Can you work these out from the model? Positions are in its coordinate system, mm. A direction names the side the tool comes from. Coordinates: 2 decimals unless noted, no trailing zeros. Order: outer loops, then holes, each group sorted by start corner. A loop starts at its lowest first (then second) coordinate and runs counter-clockwise, first axis right, second up. Notation, with made-up numbers: M -17,49 L 40,49 A14 cw 40,57 Z; hole C -18,36 d8. An arc over 180 degrees is marked long. Answer as a JSON object with one key per item and string values.
from build123d import *

# Parameters (mm, degrees)
F0_W     = 24
F0_H     = 68
F1_DEPTH = 8
F2_R     = 2
F3_DEPTH = 20
F4_W     = 39.3141321838
F4_H     = 5.4286047816
F4_W_2   = 14.8275513351
F5_DEPTH = 25
F6_W     = 16
F6_H     = 40.9167615801
F6_H_2   = 11.5639846772
F7_DEPTH = 25


with BuildPart() as f1:
    # F0 (on Top) → F1 (new body)
    with BuildSketch(Plane.XY):
        Rectangle(F0_W, F0_H)
    extrude(amount=F1_DEPTH)

    # F2 (on Right) → F3 (join, symmetric)
    with BuildSketch(Plane.YZ):
        with Locations((32, 2)):
            Circle(F2_R)
        with Locations((-15.5, 2)):
            Circle(F2_R)
    extrude(amount=F3_DEPTH, both=True)

    # F4 (on face) → F5 (cut)
    with BuildSketch(Plane.YZ.offset(12)):
        with BuildLine():
            ThreePointArc((30, 8), (32.8284271247, 6.8284271247), (34, 4))
            Line((34, 4), (34, 8))
            Line((34, 8), (30, 8))
        make_face()
        with Locations((7.5888540596, 2.7143023908)):
            Rectangle(F4_W, F4_H)
        with Locations((-26.5862243325, 2.7143023908)):
            Rectangle(F4_W_2, F4_H)
    extrude(amount=-F5_DEPTH, mode=Mode.SUBTRACT)

    # F6 (on face) → F7 (cut)
    with BuildSketch(Plane.XY.offset(8)):
        with Locations((0, 7.775218226)):
            Rectangle(F6_W, F6_H)
        with Locations((0, -25.0811139122)):
            Rectangle(F6_W, F6_H_2)
    extrude(amount=-F7_DEPTH, mode=Mode.SUBTRACT)


solid = f1.part
Item 1: I want a section at A-A, the plane y = 13. Write out the boundary of the cut face in (x, z), plus the area to 3 significant figures.
Answers follow:
{"outline": "M -12,5.43 L -8,5.43 L -8,8 L -12,8 Z; M 8,5.43 L 12,5.43 L 12,8 L 8,8 Z", "area": "20.6 mm^2"}
Item 2: Which directions (+Z, -Z, +X, -X, +Y, -Y) give clear straight access to the entire face, cutting with the end or side of a thin tool? Please do faces 1 (the flat face through (0, 28.234, 4)), 2 (the cylindrical face through (-15.944, 33.847, 1.234)), 3 (the flat face through (3, -32, 5.429)).
Answers follow:
{"face 1": "+Z, -Z", "face 2": "-X", "face 3": "-Z, +X, -X, -Y"}
Item 3: I want a section at D-D, the plane x = 9.5. Write out the boundary of the cut face in (y, z).
Answers follow:
{"outline": "M -34,5.43 L -19.17,5.43 L -19.17,0 L -12.07,0 L -12.07,5.43 L 27.25,5.43 L 27.25,0 L 34,0 L 34,4 A4 ccw 30,8 L -34,8 Z"}
Item 4: I'm going to push flat-ended pins straight in: pin 1 (16.5 mm diameter, centred on x = 0.5, y = -27.5, fed in from -Z); pin 2 (2.5 mm diameter, centred on y = 7.5, z = 4.5, fed in from +X); pin 3 (3 mm diameter, centred on x = 10.5, z = 3, fed in from -Y); pin 4 (1.5 mm diameter, centred on x = 5, z = 5, fed in from -Y). Where does each tip first touch, or does it pass through?
Answers follow:
{"pin 1": "stops at z = 5.43", "pin 2": "stops at x = 12", "pin 3": "stops at y = -19.17", "pin 4": "stops at y = -34"}
Item 5: I want a section at C-C, the plane z = 6.5. Write out the boundary of the cut face in (x, y), plus the area to 3 significant figures.
Answers follow:
{"outline": "M -12,-34 L 12,-34 L 12,33.12 L -12,33.12 Z; hole M -8,-30.86 L 8,-30.86 L 8,-19.3 L -8,-19.3 Z; hole M -8,-12.68 L 8,-12.68 L 8,28.23 L -8,28.23 Z", "area": "771 mm^2"}
Item 6: I want a section at B-B, the plane x = 1.5. Write out the boundary of the cut face in (y, z).
Answers follow:
{"outline": "M -34,5.43 L -30.86,5.43 L -30.86,8 L -34,8 Z; M -19.3,5.43 L -19.17,5.43 L -19.17,0 L -12.68,0 L -12.68,8 L -19.3,8 Z; M 28.23,0 L 34,0 L 34,4 A4 ccw 30,8 L 28.23,8 Z"}
Item 7: Please list where these lines run through material, in increasing order: line 1 (X direction, y = 19.5, z = 6); line 2 (Y direction, x = 9.5, z = 1.5); line 3 (Z direction, x = -8.5, y = -24).
Answers follow:
{"line 1": "x = -12 to -8, 8 to 12", "line 2": "y = -19.17 to -12.07, 27.25 to 34", "line 3": "z = 5.43 to 8"}
Item 8: If we mould it in two halves opening along Y, with no side actions, what happens to faces 4 (the flat face through (20, 32, 2)), 5 (the cylindrical face through (0.168, 32.797, 6.859)), 6 (the flat face through (0, -19.172, 3)), 7 (the flat face through (0, -12.683, 4))? For each: pulls with the +Y half, pulls with the -Y half, needs draft (parallel to the pull), parting line crosses it, or undercut.
Answers follow:
{"face 4": "needs draft", "face 5": "pulls with the +Y half", "face 6": "pulls with the -Y half", "face 7": "undercut"}
